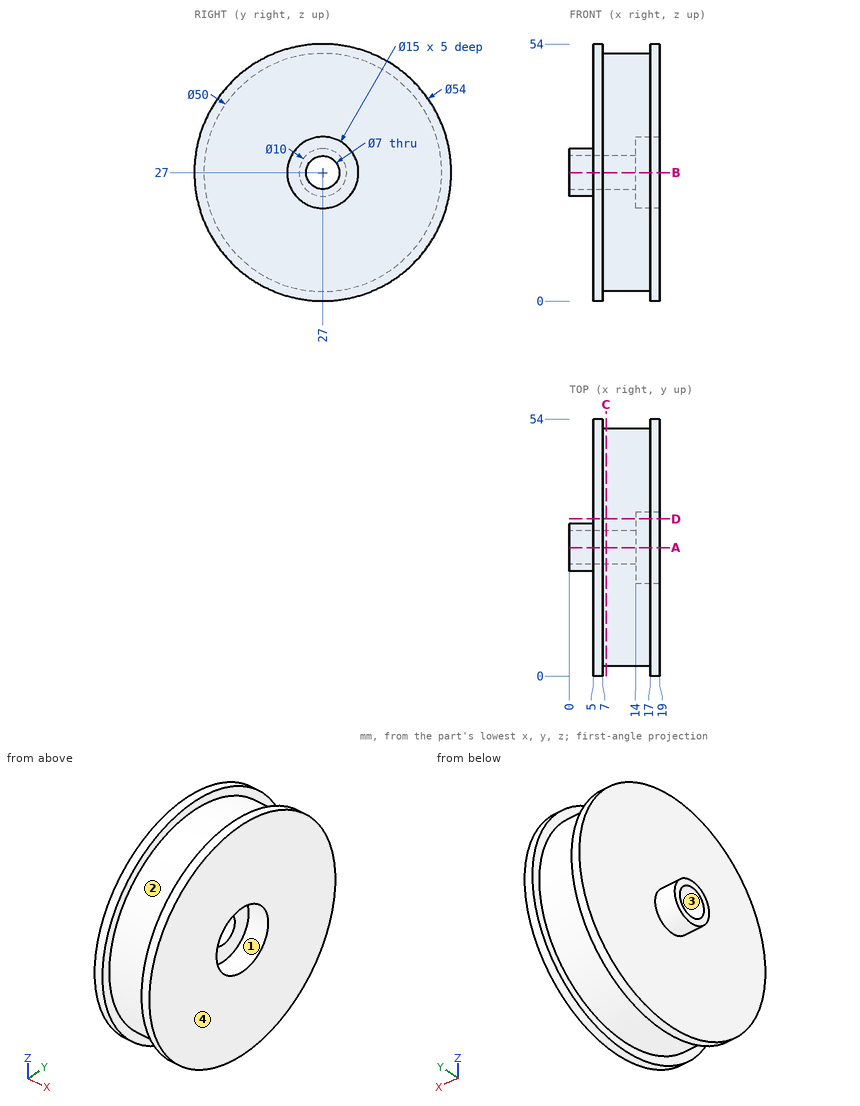
Study the drawing (mm; zero at the part's minimum x, y, z) and answer. Give positions to 0.01 mm unless a question says otherwise; leave off trailing zeros. Order: outer loops, then holes, each group sorted by start corner. A loop starts at its lowest first (then second) coordinate and runs counter-clockwise, first axis right, second up. Notation, with made-up numbers: (-39.75, 66.25) - (18.25, 66.25) arc R27 cw to (18.25, 83.25) - close; hole circle Ø3 at (-35, 48). An arc over 180 degrees is marked (long way). Use one line per item in the form item = value. Start each with the question number.
(1) A cutting plane is placed at C-C, the plane x = 7.75. Write down the section's boundary in (y, z), then the cut area to 3 significant figures.
(2) A cutting plane is placed at A-A, the plane y = 27. Write down the section's boundary in (x, z).
(3) Flat-ended cylindrical pins translate along their axes: pin 1 Ø19.5 at (y, z) = (27, 27) entering from +X; pin 2 Ø10 at (x, y) = (8, 34.5) entering from -Z; pin 3 Ø1 at (x, z) = (15.5, 37) entering from -Y; pin 4 Ø3 at (x, y) = (16.5, 14) entering from -Z. Find the tip coordinate at first contact, or state that the pin passes through.
(4) A cutting plane is placed at D-D, the plane y = 33. Write down the section's boundary in (x, z).
(5) The mould has two halves that part along Z. Classify the marked faces 1, 2, 3 and 4: released by +Z, released by -Z, zero draft, split by the parting line, or undercut.
(6) Consider line 1 (Y direction, x = 16.3, z = 27); line 2 (Z direction, x = 4, y = 27); line 3 (Y direction, x = 17.4, z = 27). Determine where each line is inside the solid, lowest interval first. Write a range as from..to.
Ans:
q1.outline = circle Ø50 at (27, 27); hole circle Ø7 at (27, 27)
q1.area = 1,930 mm^2
q2.outline = (0, 22) - (5, 22) - (5, 0) - (7, 0) - (7, 2) - (17, 2) - (17, 0) - (19, 0) - (19, 19.5) - (14, 19.5) - (14, 23.5) - (0, 23.5) - close; (0, 30.5) - (14, 30.5) - (14, 34.5) - (19, 34.5) - (19, 54) - (17, 54) - (17, 52) - (7, 52) - (7, 54) - (5, 54) - (5, 32) - (0, 32) - close
q3.pin_1 = 19
q3.pin_2 = 0.13
q3.pin_3 = 3.88
q3.pin_4 = 2.61
q4.outline = (5, 0.68) - (7, 0.68) - (7, 2.73) - (17, 2.73) - (17, 0.68) - (19, 0.68) - (19, 22.5) - (14, 22.5) - (14, 31.5) - (19, 31.5) - (19, 53.32) - (17, 53.32) - (17, 51.27) - (7, 51.27) - (7, 53.32) - (5, 53.32) - close
q5.face_1 = undercut
q5.face_2 = split by the parting line
q5.face_3 = undercut
q5.face_4 = zero draft
q6.line_1 = 2..19.5, 34.5..52
q6.line_2 = 22..23.5, 30.5..32
q6.line_3 = 0..19.5, 34.5..54
